Check sheet for the modelled part. Datum: model origin and axes. Units: mm. Face numbers are marked on the shaded views. A direction names the side the tool comes from. Give positions to 0.01 mm unless a question says otherwise; leave off trailing zeros. Loops run counter-clockwise (first coordinate to the right, second up) from the corner with the lowest first, then second, coordinate; pieces in that order, holes last. Notation, with made-up numbers: M 56.25,2.5 L 96.25,2.5 A24 ccw 96.25,40.5 Z; hole C -5.5,18.25 d9. An arc over 180 degrees is marked long. Put each result on its own line as item: value. Start each with the question number.
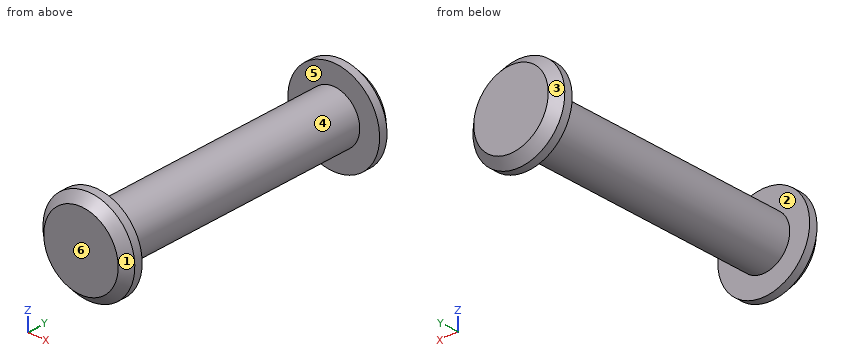
```python
from build123d import *

# Parameters (mm, degrees)
F2_SIZE = 2


with BuildPart() as f1:
    # F0 (on Right) → F1 (revolve)
    with BuildSketch(Plane.YZ):
        Polygon((-33.866643, 10.595746), (-33.866643, 0), (0, 0), (33.866643, 0), (33.866643, 10.595746), (30, 10.595746), (30, 6), (0, 6), (-30, 6), (-30, 10.595746), align=None)
    revolve(axis=Axis((0, -16.933322, 0), (0, -1, 0)))

    # F2
    f2_edges = [f1.edges().sort_by_distance(p)[0] for p in [
        (0, -33.866643, -10.595746),
        (0, 33.866643, -10.595746),
    ]]
    chamfer(f2_edges, length=F2_SIZE)


solid = f1.part
```
Q1. Access from +Z, -Z, +X, -X, +Y, -Y to the whole of each face (thin tool, end or side, straight path). Record for the marked faces 1 and 2.
Q2. Section check B-B, the plane x = 0. Record the cut outline in (y, z).
Q3. Section check A-A, the plane z = 0. Record the cut outline in (x, y).
Q4. Mould release check, pull along Y, two halves, no side actions. Record for the marked faces 3, 4, 5 and 6: pulls with the +Y half, pulls with the -Y half, needs draft (parallel to the pull), parting line crosses it, or undercut.
Q5. Section check C-C, the plane y = 17. Record the cut outline in (x, z).
Q6. Depth check by flat-ended pin: P1, Ø1, axis at x = 4, y = -9, coming from the +Z side; P2, Ø4, axis at y = -8, z = -3.5, coming from the -X side; P3, Ø2, axis at x = 0.5, y = -26, coming from the -Z side. Enter the tip coordinate at first touch or a pass-through.
Q7. Thickness scan on line 1 along Y through (x, z) = (-8, -1.25); line 2 along Y through (x, z) = (-9.25, -1.5); line 3 along X through (y, z) = (-11, 4). Record the ranges inside material, lowest first. Write a range as [from, to].
Found:
1. face 1: -Y
1. face 2: none
2. outline: M -33.87,-8.6 L -31.87,-10.6 L -30,-10.6 L -30,-6 L 30,-6 L 30,-10.6 L 31.87,-10.6 L 33.87,-8.6 L 33.87,8.6 L 31.87,10.6 L 30,10.6 L 30,6 L -30,6 L -30,10.6 L -31.87,10.6 L -33.87,8.6 Z
3. outline: M -10.6,-31.87 L -8.6,-33.87 L 8.6,-33.87 L 10.6,-31.87 L 10.6,-30 L 6,-30 L 6,30 L 10.6,30 L 10.6,31.87 L 8.6,33.87 L -8.6,33.87 L -10.6,31.87 L -10.6,30 L -6,30 L -6,-30 L -10.6,-30 Z
4. face 3: pulls with the +Y half
4. face 4: undercut
4. face 5: undercut
4. face 6: pulls with the -Y half
5. outline: C 0,0 d12
6. P1: stops at z = 4.87
6. P2: stops at x = -5.81
6. P3: stops at z = -6
7. line 1: y = [-33.87, -30], [30, 33.87]
7. line 2: y = [-33.09, -30], [30, 33.09]
7. line 3: x = [-4.47, 4.47]
